Can you work these out from the model? Positions are in its coordinate system, mm. A direction names the side the tool comes from. Coordinates: 2 decimals unless noted, no trailing zeros. Order: outer loops, then holes, each group sorted by start corner. A loop starts at its lowest first (then second) coordinate and runs counter-clockwise, first axis right, second up. Notation, with made-up numbers: (82.5, 24.5) -> (107.5, 24.5) arc R30 ccw to (107.5, 58.5) -> close; hole circle Ø9 at (74.25, 11.25). An arc over 180 degrees is marked (long way). Answer in a Markdown table with one row per item. Add a question column.
1. Imagine slicing it at C-C on y = -5. Write out the boundary of the cut face in (x, z), plus the area to 3 significant figures.
2. Imagine slicing it at D-D on z = 21. Write out the boundary of the cut face in (x, y).
3. We'd pull the mould along X, two halves only. Please class faces 4 (the face through (-9.5, -25, 13)), 5 (the face through (0, -26.5, 10)), 6 (the face through (0, -2, 25)): pulls with the +X half, pulls with the -X half, needs draft (parallel to the pull), parting line crosses it, or undercut.
4. Imagine slicing it at B-B on x = 0. Write out the boundary of the cut face in (y, z).
5. Will these pins go through, and if not, where does the flat tip stop? pin 1 (12 mm diameter, centred on x = -15.5, z = 8, fed in from +Y); pin 2 (4 mm diameter, centred on x = -16.5, z = 20.5, fed in from -Y); pin 3 (21 mm diameter, centred on x = 6.5, y = 5, fed in from -Z).
6. If I drill on line 1 along X through (y, z) = (0, 8); line 2 along X through (y, z) = (-23, 1.75); line 3 along Y through (x, z) = (0, 8), over which ranges is the centre line in solid material (lowest first)? Write a range as [from, to].
7. On a 3-axis mill with a long thin cutter (end or side, diameter ignored), from which of +Z, -Z, +X, -X, +Y, -Y can I reach the whole of each face in a straight line? I mean faces 1 (the face through (9.5, -25, 13)), 2 (the face through (0.896, 23.483, 12.325)), 3 (the face through (0, -2, 20)). Say none if no direction works.
8. Imagine slicing it at A-A on z = 3. Write out the boundary of the cut face in (x, y).
from build123d import *

# Parameters (mm, degrees)
F0_R     = 23.5
F1_DEPTH = 25
F2_W     = 19
F2_H     = 10
F3_DEPTH = 25
F5_DEPTH = 20


# Not quite as in the source:
# - a feature names something its author has since deleted; it is built from what else it names


with BuildPart() as f1:
    # F0 (on Top) → F1 (new body)
    with BuildSketch(Plane.XY):
        Circle(F0_R)
    extrude(amount=F1_DEPTH)

    # F2 (on face) → F3 (join)
    with BuildSketch(Plane.XY.offset(25)):
        with Locations((0, -23.5)):
            Rectangle(F2_W, F2_H)
    extrude(amount=-F3_DEPTH)

    # F4 (on Top) → F5 (cut)
    with BuildSketch(Plane.XY):
        with BuildLine():
            Line((-0.1196338324, -26.5), (-0.094803203, -20.9997860073))
            ThreePointArc((-0.094803203, -20.9997860073), (-3.6604096567, -20.6785251202), (-7.1196338324, -19.7562854325))
            Line((-7.1196338324, -19.7562854325), (-7.1196338324, -26.5))
            Line((-7.1196338324, -26.5), (-0.1196338324, -26.5))
        make_face()
        with BuildLine():
            ThreePointArc((6.8803661676, -19.8408810641), (3.4419080977, -20.7160147868), (-0.094803203, -20.9997860073))
            Line((-0.094803203, -20.9997860073), (-0.1196338324, -26.5))
            Line((-0.1196338324, -26.5), (6.8803661676, -26.5))
            Line((6.8803661676, -26.5), (6.8803661676, -19.8408810641))
        make_face()
        with BuildLine():
            ThreePointArc((-7.1196338324, -19.7562854325), (-3.6604096567, -20.6785251202), (-0.094803203, -20.9997860073))
            ThreePointArc((-0.094803203, -20.9997860073), (3.4419080977, -20.7160147868), (6.8803661676, -19.8408810641))
            ThreePointArc((6.8803661676, -19.8408810641), (17.1097587581, -12.1760484247), (21, 0))
            ThreePointArc((21, 0), (-12.0724415409, 17.1830193866), (-7.1196338324, -19.7562854325))
        make_face()
    extrude(amount=F5_DEPTH, mode=Mode.SUBTRACT)


solid = f1.part
Answers follow:
| question | item | result |
|---|---|---|
| 1 | outline | (-22.96, 0) -> (-20.4, 0) -> (-20.4, 20) -> (20.4, 20) -> (20.4, 0) -> (22.96, 0) -> (22.96, 25) -> (-22.96, 25) -> close |
| 1 | area | 332 mm² |
| 2 | outline | (-9.5, -28.5) -> (9.5, -28.5) -> (9.5, -21.49) arc R23.5 ccw (long way) to (-9.5, -21.49) -> close |
| 3 | face 4 | pulls with the -X half |
| 3 | face 5 | undercut |
| 3 | face 6 | needs draft |
| 4 | outline | (-28.5, 0) -> (-26.5, 0) -> (-26.5, 20) -> (21, 20) -> (21, 0) -> (23.5, 0) -> (23.5, 25) -> (-28.5, 25) -> close |
| 5 | pin 1 | stops at y = 21.49 |
| 5 | pin 2 | stops at y = -18.49 |
| 5 | pin 3 | stops at z = 20 |
| 6 | line 1 | x = [-23.5, -21], [21, 23.5] |
| 6 | line 2 | x = [-9.5, -7.12], [6.88, 9.5] |
| 6 | line 3 | y = [-28.5, -26.5], [21, 23.5] |
| 7 | face 1 | +Z, -Z, +X, -Y |
| 7 | face 2 | +Z, -Z |
| 7 | face 3 | -Z |
| 8 | outline | (-9.5, -28.5) -> (9.5, -28.5) -> (9.5, -21.49) arc R23.5 ccw (long way) to (-9.5, -21.49) -> close; hole (-7.12, -26.5) -> (6.88, -26.5) -> (6.88, -19.84) arc R21 ccw (long way) to (-7.12, -19.76) -> close |
